from build123d import *

# Parameters (mm, degrees)
F1_DEPTH = 203.2
F2_W     = 355.6
F2_H     = 19.05
F3_DEPTH = 266.7
F4_SIZE  = 6.35
F5_R     = 3.175
F6_W     = 304.8
F6_H     = 444.5
F7_DEPTH = 15.875
F8_DEPTH = 12.7


with BuildPart() as f1:
    # F0 (on Top) → F1 (new body)
    with BuildSketch(Plane.XY):
        Polygon((0, 463.55), (0, 0), (19.05, 0), (19.05, 444.5), (323.85, 444.5), (323.85, 0), (342.9, 0), (342.9, 463.55), align=None)
    extrude(amount=F1_DEPTH)

    # F2 (on Top) → F3 (join)
    with BuildSketch(Plane.XY):
        with Locations((171.45, -9.525)):
            Rectangle(F2_W, F2_H)
    extrude(amount=F3_DEPTH)

    # F4
    f4_edges = [f1.edges().sort_by_distance(p)[0] for p in [
        (171.45, -19.05, 266.7),
    ]]
    chamfer(f4_edges, length=F4_SIZE)

    # F5
    f5_edges = [f1.edges().sort_by_distance(p)[0] for p in [
        (-6.35, -19.05, 130.175),
        (-6.35, 0, 133.35),
        (171.45, 0, 0),
        (171.45, -19.05, 0),
        (0, 231.775, 0),
        (19.05, 222.25, 0),
        (171.45, 463.55, 0),
        (171.45, 444.5, 0),
        (323.85, 222.25, 0),
        (342.9, 231.775, 0),
        (349.25, 0, 133.35),
        (349.25, -19.05, 130.175),
        (19.05, 222.25, 203.2),
        (171.45, 444.5, 203.2),
        (323.85, 222.25, 203.2),
        (-6.35, -9.525, 0),
        (349.25, -9.525, 0),
        (346.075, 0, 0),
        (-3.175, 0, 0),
        (171.45, 0, 266.7),
    ]]
    fillet(f5_edges, radius=F5_R)

    # F6 (on Top) → F7 (join)
    with BuildSketch(Plane.XY):
        with Locations((171.45, 222.25)):
            Rectangle(F6_W, F6_H)
    extrude(amount=F7_DEPTH)

    # F6 (on Top) → F8 (cut)
    with BuildSketch(Plane.XY):
        with Locations((171.45, 222.25)):
            Rectangle(F6_W, F6_H)
    extrude(amount=F8_DEPTH, mode=Mode.SUBTRACT)


solid = f1.part
Can you work these out from the model? Positions are in its coordinate system, mm. A direction names the side the tool comes from. Give positions to 0.01 mm unless a question says otherwise; leave off trailing zeros. Loops run counter-clockwise (first coordinate to the right, second up) from the corner with the lowest first, then second, coordinate; pieces in that order, holes last. Notation, with made-up numbers: M 19.5,-13 L 60.5,-13 A24 ccw 60.5,7 Z; hole C 52.25,-13 d5. An arc over 180 degrees is marked long. One line per item, written item: value. Start each with the question number.
1) On a 3-axis mill with a long thin cutter (end or side, diameter ignored), from which of +Z, -Z, +X, -X, +Y, -Y can I reach the whole of each face in a straight line? I mean faces 1 (the face through (323.85, 225, 107)), 2 (the face through (342.9, 229, 102)), 3 (the face through (171, 456, 203.2)), 4 (the face through (174, 463.55, 102)). Say none if no direction works.
2) If we section it at C-C, the plane z = 236.5: Write out the boundary of the cut face in (x, y) (3 decimals), and give its area (3 significant figures).
3) Thinking about a two-plate mould opening in Y: for faces 5 (the face through (169, 225, 12.7)), 6 (the face through (169, 444.5, 107)), 7 (the face through (169, -19.05, 130)), 8 (the face through (0, 235, 102)), which applies, +Y half, -Y half, draft (parallel to the pull), parting line (faces both ways), or undercut?
4) If we section it at B-B, the plane y = 296: Write out the boundary of the cut face in (x, z) (3 decimals).
5) If we section it at D-D, the plane x = 156: Write out the boundary of the cut face in (y, z) (3 decimals), and give its area (3 significant figures).
6) I'm going to push flat-ended pins straight in: pin 1 (10 mm diameter, centred on y = 123.5, z = 180, fed in from +X); pin 2 (10.5 mm diameter, centred on y = 177.5, z = 6.5, fed in from -X); pin 3 (1 mm diameter, centred on x = 255.5, z = 222, fed in from +Y). Where does each tip first touch, or does it pass through?
7) If we section it at A-A, the plane z = 71: Write out the boundary of the cut face in (x, y) (3 decimals).
8) If I drill on line 1 (X direction, y = 77.5, z = 67.5); line 2 (Y direction, x = 106.5, z = 29); line 3 (Z direction, x = 97.5, y = 9.5) (3 decimals), over which ranges is the centre line in solid material (lowest first)? Write a range as [from, to].
Completed:
1. face 1: +Z
1. face 2: +Z, -Z, +X, +Y
1. face 3: +Z, +X, -X, +Y
1. face 4: +Z, -Z, +X, -X, +Y
2. outline: M -6.35,-15.875 A3.175 ccw -3.175,-19.05 L 346.075,-19.05 A3.175 ccw 349.25,-15.875 L 349.25,-3.175 A3.175 ccw 346.075,0 L -3.175,0 A3.175 ccw -6.35,-3.175 Z
2. area: 6,770 mm^2
3. face 5: undercut
3. face 6: undercut
3. face 7: -Y half
3. face 8: draft
4. outline: M 0,3.175 A3.175 ccw 3.175,0 L 15.875,0 A3.175 ccw 19.05,3.175 L 19.05,12.7 L 323.85,12.7 L 323.85,3.175 A3.175 ccw 327.025,0 L 339.725,0 A3.175 ccw 342.9,3.175 L 342.9,203.2 L 327.025,203.2 A3.175 ccw 323.85,200.025 L 323.85,15.875 L 19.05,15.875 L 19.05,200.025 A3.175 ccw 15.875,203.2 L 0,203.2 Z
5. outline: M -19.05,3.175 A3.175 ccw -15.875,0 L -3.175,0 A3.175 ccw 0,3.175 L 0,12.7 L 444.5,12.7 L 444.5,3.175 A3.175 ccw 447.675,0 L 460.375,0 A3.175 ccw 463.55,3.175 L 463.55,203.2 L 447.675,203.2 A3.175 ccw 444.5,200.025 L 444.5,15.875 L 0,15.875 L 0,263.525 A3.175 ccw -3.175,266.7 L -12.7,266.7 L -19.05,260.35 Z
5. area: 10,300 mm^2
6. pin 1: stops at x = 342.9
6. pin 2: stops at x = 0
6. pin 3: stops at y = 0
7. outline: M -6.35,-15.875 A3.175 ccw -3.175,-19.05 L 346.075,-19.05 A3.175 ccw 349.25,-15.875 L 349.25,-3.175 A3.175 ccw 346.075,0 L 342.9,0 L 342.9,463.55 L 0,463.55 L 0,0 L -3.175,0 A3.175 ccw -6.35,-3.175 Z; hole M 19.05,0 L 323.85,0 L 323.85,444.5 L 19.05,444.5 Z
8. line 1: x = [0, 19.05], [323.85, 342.9]
8. line 2: y = [-19.05, 0], [444.5, 463.55]
8. line 3: z = [12.7, 15.875]
